Geometry check sheet. Reference: the model listing, model coordinates, mm. A direction names the side the tool comes from. Coordinates: 2 decimals unless noted, no trailing zeros. Order: outer loops, then holes, each group sorted by start corner. A loop starts at its lowest first (then second) coordinate and runs counter-clockwise, first axis right, second up. Notation, with made-up numbers: M 5.25,66.25 L 31.25,66.25 A20 cw 31.25,92.25 Z; hole C 50.5,59 d7. An arc over 180 degrees is marked long. One line per item, written item: value. Start each with the question number.
1) Sectioned sample at B-B, the plane x = 0. Enter the section's corners in (y, z), then the cut area to 3 significant figures.
2) Sectioned sample at D-D, the plane z = 19. Enter the section's corners in (x, y), then the cut area to 3 significant figures.
3) Sectioned sample at A-A, the plane y = -26.5. Enter the section's corners in (x, z), then the cut area to 3 significant figures.
4) Access from +Z, -Z, +X, -X, +Y, -Y to the whole of each face (thin tool, end or side, straight path). Record for faces 4 (the cylindrical face through (14.782, -44.264, -28.885)), 5 (the flat face through (0, -44, -26.337)), 6 (the flat face through (-14.614, -13, 12)).
5) Go/stop test with flat-tipped pins: P1, Ø6, axis at x = 5, y = -30.5, coming from the +Z side; P2, Ø17.5, axis at x = 10.5, z = 10, coming from the -Y side; P3, Ø12, axis at x = -24.5, y = -36, coming from the +Z side; P4, Ø13.5, axis at x = 0, z = 31.51, coming from the +Y side. Record where each tip stops, or that it passes through.
6) Sectioned sample at C-C, the plane y = -15. Enter the section's corners in (x, z).
7) Thickness scan on L1, parallel to Z at x = 0, y = -36.25; L2, parallel to Z at x = 0, y = -16.25; L3, parallel to Z at x = -5, y = -54. Record the ranges inside material, lowest first. Write a range as from..to.
8) Draft check along Z on faces 1 (the flat face through (14.614, -13, 12)), 2 (the cylindrical face through (-1.902, -37.594, 45.996)), 3 (the cylindrical face through (20.21, -12.52, -21.03)). Enter one of: pulls with the +Z half, pulls with the -Z half, needs draft (parallel to the pull), parting line crosses it, or undercut.
```python
from build123d import *

# Parameters (mm, degrees)
F0_W     = 29.2275138199
F0_H     = 23.781274911
F1_DEPTH = 25.4
F2_R     = 14.61375691
F2_R_2   = 7.4161763195
F3_DEPTH = 17.018
F4_W     = 66.4506405592
F4_H     = 5.1697115414
F5_DEPTH = 36.83
F6_R     = 12.7
F7_R     = 7.792205292
F8_DEPTH = 5.1707115414
F9_DEPTH = 19.812


with BuildPart() as f1:
    # F0 (on Front) → F1 (new body)
    with BuildSketch(Plane.XZ):
        with BuildLine():
            Line((7.4161763195, 31.5062142909), (14.61375691, 31.5062142909))
            ThreePointArc((14.61375691, 31.5062142909), (0, 46.1199712008), (-14.61375691, 31.5062142909))
            Line((-14.61375691, 31.5062142909), (-7.4161763195, 31.5062142909))
            ThreePointArc((-7.4161763195, 31.5062142909), (0, 38.9223906104), (7.4161763195, 31.5062142909))
        make_face()
        with BuildLine():
            Line((14.61375691, -7.7249393798), (14.61375691, -31.5062142909))
            Line((14.61375691, -31.5062142909), (33.2253202796, -31.5062142909))
            Line((33.2253202796, -31.5062142909), (33.2253202796, -26.3365027495))
            ThreePointArc((33.2253202796, -26.3365027495), (20.0649576124, -20.885302047), (14.61375691, -7.7249393798))
        make_face()
        with BuildLine():
            Line((-14.61375691, -7.7249393798), (14.61375691, -7.7249393798))
            Line((14.61375691, -7.7249393798), (14.61375691, 31.5062142909))
            ThreePointArc((14.61375691, 31.5062142909), (0, 16.8924573809), (-14.61375691, 31.5062142909))
            Line((-14.61375691, 31.5062142909), (-14.61375691, -7.7249393798))
        make_face()
        with BuildLine():
            Line((-33.2253202796, -31.5062142909), (-14.61375691, -31.5062142909))
            Line((-14.61375691, -31.5062142909), (-14.61375691, -7.7249393798))
            ThreePointArc((-14.61375691, -7.7249393798), (-20.0649576124, -20.885302047), (-33.2253202796, -26.3365027495))
            Line((-33.2253202796, -26.3365027495), (-33.2253202796, -31.5062142909))
        make_face()
        with BuildLine():
            ThreePointArc((-14.61375691, 31.5062142909), (0, 16.8924573809), (14.61375691, 31.5062142909))
            Line((14.61375691, 31.5062142909), (7.4161763195, 31.5062142909))
            ThreePointArc((7.4161763195, 31.5062142909), (0, 24.0900379714), (-7.4161763195, 31.5062142909))
            Line((-7.4161763195, 31.5062142909), (-14.61375691, 31.5062142909))
        make_face()
        with Locations((0, -19.6155768353)):
            Rectangle(F0_W, F0_H)
    extrude(amount=F1_DEPTH)

    # F2 (on face) → F3 (join)
    with BuildSketch(Plane.XZ.offset(25.4)):
        with Locations((0, 31.5062142909)):
            Circle(F2_R)
        with Locations((0, 31.5062142909)):
            Circle(F2_R_2, mode=Mode.SUBTRACT)
    extrude(amount=F3_DEPTH)

    # F4 (on face) → F5 (join)
    with BuildSketch(Plane.XZ.offset(25.4)):
        with Locations((0, -28.9213585202)):
            Rectangle(F4_W, F4_H)
    extrude(amount=F5_DEPTH)

    # F6
    f6_edges = [f1.edges().sort_by_distance(p)[0] for p in [
        (-33.22532, -62.23, -28.921359),
        (33.22532, -62.23, -28.921359),
    ]]
    fillet(f6_edges, radius=F6_R)

    # F7 (on face) → F8 (cut, through all)
    with BuildSketch(Plane.XY.offset(-26.3365027495)):
        with Locations((-20.5253202796, -49.53)):
            Circle(F7_R)
        with Locations((20.5253202796, -49.53)):
            Circle(F7_R)
    extrude(amount=-F8_DEPTH, mode=Mode.SUBTRACT)

    # F9 (add, through all): a face of the model
    f9_faces = [f1.faces().sort_by_distance(p)[0] for p in [
        (-14.2004174456, -42.418, 31.5062142909),
    ]]
    extrude(f9_faces, amount=F9_DEPTH)


solid = f1.part
```
Final values:
1. outline: M -62.23,-31.51 L 0,-31.51 L 0,24.09 L -62.23,24.09 L -62.23,16.89 L -25.4,16.89 L -25.4,-26.34 L -62.23,-26.34 Z; M -62.23,38.92 L 0,38.92 L 0,46.12 L -62.23,46.12 Z
1. area: 2,320 mm^2
2. outline: M -14.61,-25.4 L -7.56,-25.4 L -7.56,-62.23 L 7.56,-62.23 L 7.56,-25.4 L 14.61,-25.4 L 14.61,0 L -14.61,0 Z
2. area: 1,300 mm^2
3. outline: M -33.23,-31.51 L 33.23,-31.51 L 33.23,-26.34 L -33.23,-26.34 Z; C 0,31.51 d29.23; hole C 0,31.51 d14.83
3. area: 842 mm^2
4. face 4: -Z
4. face 5: +X, -X, -Y
4. face 6: +Z, -X, +Y, -Y
5. P1: stops at z = 45.98
5. P2: stops at y = -25.4
5. P3: stops at z = -26.34
5. P4: passes through
6. outline: M -33.23,-31.51 L 33.23,-31.51 L 33.23,-26.34 A18.61 cw 14.61,-7.72 L 14.61,31.51 A14.61 ccw -14.61,31.51 L -14.61,-7.72 A18.61 cw -33.23,-26.34 Z; hole C 0,31.51 d14.83
7. L1: z = -31.51..-26.34, 16.89..24.09, 38.92..46.12
7. L2: z = -31.51..24.09, 38.92..46.12
7. L3: z = -31.51..-26.34, 17.77..26.03, 36.98..45.24
8. face 1: needs draft
8. face 2: undercut
8. face 3: pulls with the +Z half
